Source: CAD feature listing. Evaluate the final solid. Frame: model axes, mm. A direction names the side the tool comes from. Coordinates: 2 decimals unless noted, no trailing zeros. Loops run counter-clockwise (first coordinate to the right, second up) from the corner with the lowest first, then second, coordinate; pieces in that order, holes last.
```python
from build123d import *

# Parameters (mm, degrees)
SKETCH2_W                          = 65
SKETCH2_H                          = 100
BOSS_EXTRUDE1_DEPTH                = 4.5
F_36_0_1065_DIAMETER_HOLE1_D       = 2.7051
FILLET1_R                          = 5
TAP_DRILL_FOR_M2_2_HELICOIL1_D     = 2.3
TAP_DRILL_FOR_M2_2_HELICOIL1_DEPTH = 4.5
TAP_DRILL_FOR_M2_2_HELICOIL1_TIP   = 0.690989712
SKETCH14_W                         = 7
SKETCH14_H                         = 4
CUT_EXTRUDE1_DEPTH                 = 10
SKETCH16_R                         = 13
CUT_EXTRUDE2_DEPTH                 = 17


with BuildPart() as part:
    # Sketch2 → Boss-Extrude1 (new body)
    with BuildSketch(Plane(origin=(0, 0, 0), x_dir=(1, 0, 0), z_dir=(0, 1, 0))):
        Rectangle(SKETCH2_W, SKETCH2_H)
    extrude(amount=BOSS_EXTRUDE1_DEPTH)

    # #36 (0.1065) Diameter Hole1 (through all)
    with Locations(Plane(origin=(0, 4.5, 0), x_dir=(1, 0, 0), z_dir=(0, 1, 0))):
        with Locations((-26.15, 43.65), (26.15, 43.65), (26.15, -43.65), (-26.15, -43.65)):
            Hole(F_36_0_1065_DIAMETER_HOLE1_D / 2)

    # Fillet1
    fillet1_edges = [part.edges().sort_by_distance(p)[0] for p in [
        (32.5, 2.25, 50),
        (-32.5, 2.25, 50),
        (-32.5, 2.25, -50),
        (32.5, 2.25, -50),
    ]]
    fillet(fillet1_edges, radius=FILLET1_R)

    # Tap Drill for M2.2 Helicoil1
    with Locations(Plane(origin=(0, 4.5, 0), x_dir=(1, 0, 0), z_dir=(0, 1, 0))):
        with Locations((14, -32.631381325), (-14, -44.131381325)):
            Hole(TAP_DRILL_FOR_M2_2_HELICOIL1_D / 2, depth=TAP_DRILL_FOR_M2_2_HELICOIL1_DEPTH)
            with Locations((0, 0, -(TAP_DRILL_FOR_M2_2_HELICOIL1_DEPTH + TAP_DRILL_FOR_M2_2_HELICOIL1_TIP / 2))):  # 118° drill point
                Cone(0, TAP_DRILL_FOR_M2_2_HELICOIL1_D / 2, TAP_DRILL_FOR_M2_2_HELICOIL1_TIP, mode=Mode.SUBTRACT)

    # Sketch14 → Cut-Extrude1 (cut)
    with BuildSketch(Plane(origin=(0, 4.5, 0), x_dir=(1, 0, 0), z_dir=(0, 1, 0))):
        with Locations((0, -15)):
            Rectangle(SKETCH14_W, SKETCH14_H)
    extrude(amount=-CUT_EXTRUDE1_DEPTH, mode=Mode.SUBTRACT)

    # Sketch16 → Cut-Extrude2 (cut)
    with BuildSketch(Plane(origin=(0, 4.5, 0), x_dir=(1, 0, 0), z_dir=(0, 1, 0))):
        with Locations(Location((0, 14.115370647, 0), (0, 0, 270))):
            Circle(SKETCH16_R)
    extrude(amount=-CUT_EXTRUDE2_DEPTH, mode=Mode.SUBTRACT)


solid = part.part
```
Q1. Material intervals for line 1 along Z through (x, y) = (-26.15, 2.95); line 2 along X through (y, z) = (2.6, -43.65); line 3 along Z through (x, y) = (-14, 2.1), sorted ascending.
Q2. Section query A-A on x = 0. Return the cut outline in (y, z), then the cut area to 3 significant figures.
Q3. Reachability of faces 5 (the flat face through (-0.5, 0, -0.7)), 6 (the flat face through (0, 2, 13)) from +Z, -Z, +X, -X, +Y, -Y: full face, straight path, thin tool, end or side. Return the list, or none.
Q4. Section query D-D on y = 0.7. Count the separate pieces of the cut face and the enclosed holes in it, then the cut area to 3 significant figures.
Q5. Section query C-C on x = 9. Return the cut outline in (y, z), then the cut area to 3 significant figures.
Q6. Section query B-B on z = -43.65. Return the cut outline in (x, y), then the cut area to 3 significant figures.
Q7. First-contact query: pin 1 Ø3.5 at (x, z) = (-26.15, -43.65) entering from +Y. Flat tip, straight axial feed; report the tip coordinate or a pass-through.
Q8. Draft query along Z for faces 1 (the flat face through (-32.5, 2, 1)), 2 (the cylindrical face through (-31.07, 2.28, -48.5)), 3 (the cylindrical face through (31, 2.28, 48.57)), 4 (the cylindrical face through (25.53, 2.22, -42.45)). Return one class per face: released by +Z, released by -Z, zero draft, split by the parting line, or undercut.
Resolved:
1. line 1: z = -50 to -45, -42.3 to 42.3, 45 to 50
1. line 2: x = -32.5 to -27.5, -24.8 to 24.8, 27.5 to 32.5
1. line 3: z = -50 to 42.98, 45.28 to 50
2. outline: (0, -50) - (4.5, -50) - (4.5, -27.12) - (0, -27.12) - close; (0, -1.12) - (4.5, -1.12) - (4.5, 13) - (0, 13) - close; (0, 17) - (4.5, 17) - (4.5, 50) - (0, 50) - close
2. area: 315 mm2
3. face 5: +Z, -Z, +X, -X, -Y
3. face 6: +Y, -Y
4. separate pieces: 1
4. enclosed holes: 8
4. area: 5,890 mm2
5. outline: (0, -50) - (4.5, -50) - (4.5, -23.5) - (0, -23.5) - close; (0, -4.73) - (4.5, -4.73) - (4.5, 50) - (0, 50) - close
5. area: 366 mm2
6. outline: (-32.5, 0) - (-27.5, 0) - (-27.5, 4.5) - (-32.5, 4.5) - close; (-24.8, 0) - (24.8, 0) - (24.8, 4.5) - (-24.8, 4.5) - close; (27.5, 0) - (32.5, 0) - (32.5, 4.5) - (27.5, 4.5) - close
6. area: 268 mm2
7. pin 1: stops at y = 4.5
8. face 1: zero draft
8. face 2: released by -Z
8. face 3: released by +Z
8. face 4: undercut
